Job drawing, mm, ordinate dimensions from the low corner. One solid piece. Round coordinates to 2 decimals unless told otherwise and drop trailing zeros. Loops run counter-clockwise (first coordinate to the right, second up) from the corner with the lowest first, then second, coordinate; pieces in that order, holes last.
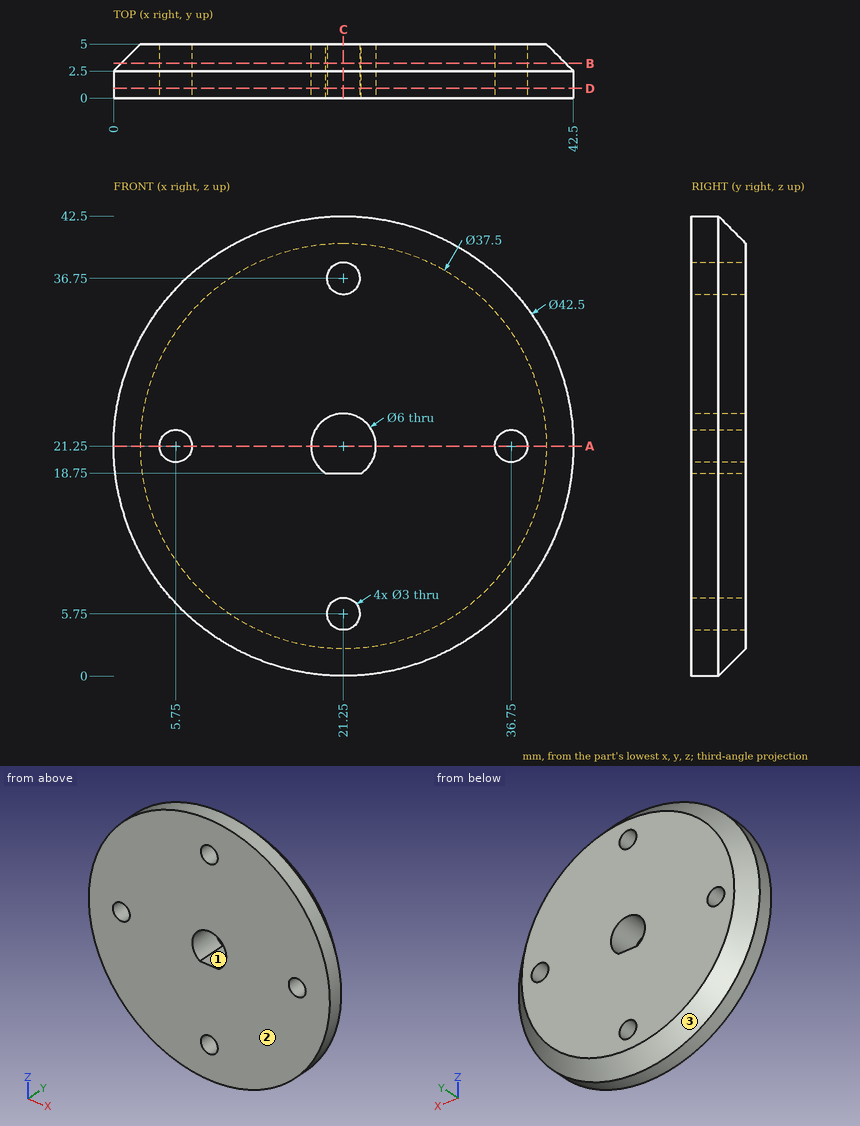
1) Wall check: line 1 along X through (y, z) = (1.5, 21.25); line 2 along Z through (x, y) = (21, 3); line 3 along Z through (x, y) = (21, 2.45). Give the ranges that are in metal, low to high.
Values:
line 1: x = 0 to 4.25, 7.25 to 18.25, 24.25 to 35.25, 38.25 to 42.5
line 2: z = 0.5 to 4.27, 7.23 to 18.75, 24.24 to 35.27, 38.23 to 42
line 3: z = 0 to 4.27, 7.23 to 18.75, 24.24 to 35.27, 38.23 to 42.5
2) Slice it at B-B, the plane y = 3.2. Give the cut face in (x, z), then the cut area to 3 significant figures.
Values:
outline: circle Ø41.1 at (21.25, 21.25); hole circle Ø3 at (5.75, 21.25); hole (19.59, 18.75) - (22.91, 18.75) arc R3 ccw (long way) to start; hole circle Ø3 at (21.25, 5.75); hole circle Ø3 at (21.25, 36.75); hole circle Ø3 at (36.75, 21.25)
area: 1,270 mm2
3) Drop flat-ended pins along their axis: pin 1 Ø1 at (x, y) = (13, 3) entering from -Z; pin 2 Ø2 at (x, y) = (11.5, 1.5) entering from +Z; pin 3 Ø2 at (x, y) = (19, 2) entering from +Z. Give the stop position or say it passes through.
Values:
pin 1: stops at z = 1.63
pin 2: stops at z = 40.61
pin 3: stops at z = 42.46
4) Slice it at A-A, the plane z = 21.25. Give the cut face in (x, y), then the cut area to 3 significant figures.
Values:
outline: (0, 0) - (4.25, 0) - (4.25, 5) - (2.5, 5) - (0, 2.5) - close; (7.25, 0) - (18.25, 0) - (18.25, 5) - (7.25, 5) - close; (24.25, 0) - (35.25, 0) - (35.25, 5) - (24.25, 5) - close; (38.25, 0) - (42.5, 0) - (42.5, 2.5) - (40, 5) - (38.25, 5) - close
area: 146 mm2
5) Mould opens along Z. For the marked faces 1, 2 and 3 say: released by +Z, released by -Z, zero draft, split by the parting line, or undercut.
Values:
face 1: undercut
face 2: zero draft
face 3: split by the parting line
6) Slice it at C-C, the plane x = 21.25. Give the cut face in (y, z), then the cut area to 3 significant figures.
Values:
outline: (0, 0) - (2.5, 0) - (5, 2.5) - (5, 4.25) - (0, 4.25) - close; (0, 7.25) - (5, 7.25) - (5, 18.75) - (0, 18.75) - close; (0, 24.25) - (5, 24.25) - (5, 35.25) - (0, 35.25) - close; (0, 38.25) - (5, 38.25) - (5, 40) - (2.5, 42.5) - (0, 42.5) - close
area: 149 mm2
7) Slice it at D-D, the plane y = 0.9. Give the cut face in (x, z), then the cut area to 3 significant figures.
Values:
outline: circle Ø42.5 at (21.25, 21.25); hole circle Ø3 at (5.75, 21.25); hole (19.59, 18.75) - (22.91, 18.75) arc R3 ccw (long way) to start; hole circle Ø3 at (21.25, 5.75); hole circle Ø3 at (21.25, 36.75); hole circle Ø3 at (36.75, 21.25)
area: 1,360 mm2
